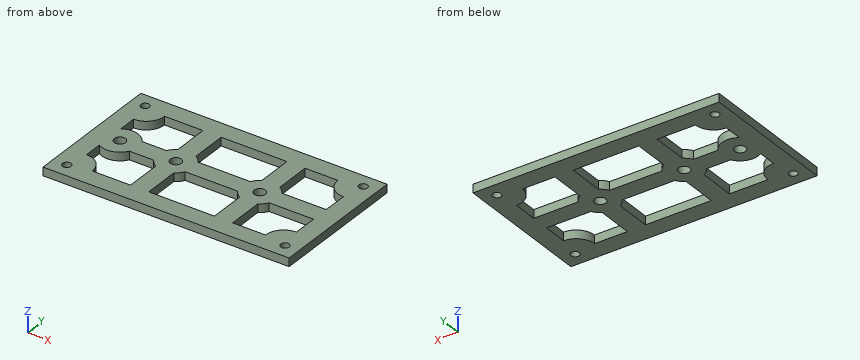
from build123d import *

# Parameters (mm, degrees)
SKETCH1_W            = 88
SKETCH1_H            = 50
BOSS_EXTRUDE1_DEPTH  = 3
SKETCH2_R            = 2
CUT_EXTRUDE1_DEPTH   = 51.695167423
SKETCH3_R            = 1.5
CUT_EXTRUDE2_DEPTH   = 51.695167423
LPATTERN1_COUNT      = 2
LPATTERN1_PITCH      = 78
LPATTERN1_COUNT_DIR2 = 2
LPATTERN1_PITCH_DIR2 = 40
CUT_EXTRUDE3_DEPTH   = 51.695167423


with BuildPart() as part:
    # Sketch1 → Boss-Extrude1 (new body)
    with BuildSketch(Plane.XY):
        Rectangle(SKETCH1_W, SKETCH1_H)
    extrude(amount=BOSS_EXTRUDE1_DEPTH)

    # Sketch2 → Cut-Extrude1 (cut, through all)
    with BuildSketch(Plane.XY.offset(3)):
        with Locations((-34, 0)):
            Circle(SKETCH2_R)
        with Locations((-14, 0)):
            Circle(SKETCH2_R)
        with Locations((16, 0)):
            Circle(SKETCH2_R)
    extrude(amount=-CUT_EXTRUDE1_DEPTH, mode=Mode.SUBTRACT)

    # Sketch3 → Cut-Extrude2 (cut, through all)
    with BuildSketch(Plane.XY.offset(3)):
        with Locations((-39, 20)):
            Circle(SKETCH3_R)
    cut_extrude2 = extrude(amount=-CUT_EXTRUDE2_DEPTH, mode=Mode.SUBTRACT)

    # LPattern1: Cut-Extrude2 2 × 2
    with Locations(*[(i * LPATTERN1_PITCH, -j * LPATTERN1_PITCH_DIR2, 0) for i in range(LPATTERN1_COUNT) for j in range(LPATTERN1_COUNT_DIR2) if (i, j) != (0, 0)]):
        add(cut_extrude2, mode=Mode.SUBTRACT)

    # Sketch4 → Cut-Extrude3 (cut, through all)
    with BuildSketch(Plane.XY.offset(3)):
        with BuildLine():
            Line((37.5, 3.25), (37.5, 12))
            ThreePointArc((37.5, 12), (32.903805922, 13.903805922), (31, 18.5))
            Line((31, 18.5), (19.25, 18.5))
            Line((19.25, 18.5), (19.25, 5.629165125))
            ThreePointArc((19.25, 5.629165125), (20.596194078, 4.596194078), (21.629165125, 3.25))
            Line((21.629165125, 3.25), (37.5, 3.25))
        make_face()
        with BuildLine():
            Line((-28.370834875, 3.25), (-19.629165125, 3.25))
            ThreePointArc((-19.629165125, 3.25), (-18.596194078, 4.596194078), (-17.25, 5.629165125))
            Line((-17.25, 5.629165125), (-17.25, 18.5))
            Line((-17.25, 18.5), (-31, 18.5))
            ThreePointArc((-31, 18.5), (-32.903805922, 13.903805922), (-37.5, 12))
            Line((-37.5, 12), (-37.5, 5.477225575))
            ThreePointArc((-37.5, 5.477225575), (-32.459393148, 6.314786657), (-28.370834875, 3.25))
        make_face()
        with BuildLine():
            Line((-8.370834875, 3.25), (10.370834875, 3.25))
            ThreePointArc((10.370834875, 3.25), (11.403805922, 4.596194078), (12.75, 5.629165125))
            Line((12.75, 5.629165125), (12.75, 18.5))
            Line((12.75, 18.5), (-10.75, 18.5))
            Line((-10.75, 18.5), (-10.75, 5.629165125))
            ThreePointArc((-10.75, 5.629165125), (-9.403805922, 4.596194078), (-8.370834875, 3.25))
        make_face()
        with BuildLine():
            Line((-28.370834875, -3.25), (-19.629165125, -3.25))
            ThreePointArc((-19.629165125, -3.25), (-18.596194078, -4.596194078), (-17.25, -5.629165125))
            Line((-17.25, -5.629165125), (-17.25, -18.5))
            Line((-17.25, -18.5), (-31, -18.5))
            ThreePointArc((-31, -18.5), (-32.903805922, -13.903805922), (-37.5, -12))
            Line((-37.5, -12), (-37.5, -5.477225575))
            ThreePointArc((-37.5, -5.477225575), (-32.459393148, -6.314786657), (-28.370834875, -3.25))
        make_face()
        with BuildLine():
            Line((37.5, -12), (37.5, -3.25))
            Line((37.5, -3.25), (21.629165125, -3.25))
            ThreePointArc((21.629165125, -3.25), (20.596194078, -4.596194078), (19.25, -5.629165125))
            Line((19.25, -5.629165125), (19.25, -18.5))
            Line((19.25, -18.5), (31, -18.5))
            ThreePointArc((31, -18.5), (32.903805922, -13.903805922), (37.5, -12))
        make_face()
        with BuildLine():
            Line((-8.370834875, -3.25), (10.370834875, -3.25))
            ThreePointArc((10.370834875, -3.25), (11.403805922, -4.596194078), (12.75, -5.629165125))
            Line((12.75, -5.629165125), (12.75, -18.5))
            Line((12.75, -18.5), (-10.75, -18.5))
            Line((-10.75, -18.5), (-10.75, -5.629165125))
            ThreePointArc((-10.75, -5.629165125), (-9.403805922, -4.596194078), (-8.370834875, -3.25))
        make_face()
    extrude(amount=-CUT_EXTRUDE3_DEPTH, mode=Mode.SUBTRACT)


solid = part.part
Geometry: final body of the model. Coordinates: model frame, mm. Coordinates: 2 decimals unless noted, no trailing zeros. Write each loop counter-clockwise with the first axis right and the second up, starting at its lowest first coordinate (ties: lowest second). Pieces come first, ordered by that corner, then holes. Notation, with made-up numbers: (83.25, 57) - (132.25, 57) arc R18 ccw to (132.25, 79) - close; hole circle Ø5 at (6, 52). An arc over 180 degrees is marked (long way). Return JSON: item names as keys, results as strings.
Item 1: Section query B-B (y = -9.5). Output: boundary loops of the cut face in (x, z).
Completed:
{"outline": "(-44, 0) - (-37.5, 0) - (-37.5, 3) - (-44, 3) - close; (-17.25, 0) - (-10.75, 0) - (-10.75, 3) - (-17.25, 3) - close; (12.75, 0) - (19.25, 0) - (19.25, 3) - (12.75, 3) - close; (37.5, 0) - (44, 0) - (44, 3) - (37.5, 3) - close"}
Item 2: Section query A-A (x = -6). Output: boundary loops of the cut face in (y, z).
Completed:
{"outline": "(-25, 0) - (-18.5, 0) - (-18.5, 3) - (-25, 3) - close; (-3.25, 0) - (3.25, 0) - (3.25, 3) - (-3.25, 3) - close; (18.5, 0) - (25, 0) - (25, 3) - (18.5, 3) - close"}
Item 3: Line query: L1, parallel to X at y = -18, z = 0.9; L2, parallel to Y at x = -39, z = 1.7; L3, parallel to Y at x = 7.5, z = 2.35. Output: solid intervals per line, ascending.
Completed:
{"L1": "x = -44 to -31.02, -17.25 to -10.75, 12.75 to 19.25, 31.02 to 44", "L2": "y = -25 to -21.5, -18.5 to 18.5, 21.5 to 25", "L3": "y = -25 to -18.5, -3.25 to 3.25, 18.5 to 25"}
Item 4: Section query D-D (x = 16.5). Output: boundary loops of the cut face in (y, z), and give its area (3 significant figures).
Completed:
{"outline": "(-25, 0) - (-1.94, 0) - (-1.94, 3) - (-25, 3) - close; (1.94, 0) - (25, 0) - (25, 3) - (1.94, 3) - close", "area": "138 mm2"}
Item 5: Pin query (flat end, axial travel): pin 1 Ø2.5 at (x, y) = (-39, 20) entering from -Z. Return the tip coordinate at first contact, or that it passes through.
Completed:
{"pin 1": "passes through"}
Item 6: Section query C-C (y = 20). Output: boundary loops of the cut face in (x, z), and give its area (3 significant figures).
Completed:
{"outline": "(-44, 0) - (-40.5, 0) - (-40.5, 3) - (-44, 3) - close; (-37.5, 0) - (37.5, 0) - (37.5, 3) - (-37.5, 3) - close; (40.5, 0) - (44, 0) - (44, 3) - (40.5, 3) - close", "area": "246 mm2"}
